For this review, take the finished solid that the model builds, in its own axes (mm). Round coordinates to 2 decimals unless told otherwise and drop trailing zeros. Write each loop counter-clockwise with the first axis right and the second up, starting at its lowest first coordinate (ties: lowest second). Pieces come first, ordered by that corner, then holes. Notation, with made-up numbers: (2.5, 0.25) -> (61.5, 0.25) arc R5 cw to (61.5, 7.25) -> close; hole circle Ø8 at (3, -5.75). An arc over 180 degrees is marked (long way). Answer in a Markdown table with one row per item.
from build123d import *

# Parameters (mm, degrees)
F0_R     = 4
F0_R_2   = 2.5
F0_R_3   = 1.5
F1_DEPTH = 3
F2_DEPTH = 3
F3_R     = 0.6
F4_R     = 2


with BuildPart() as f1:
    # F0 (on Top) → F1 (new body)
    with BuildSketch(Plane.XY):
        Circle(F0_R)
        Circle(F0_R_2, mode=Mode.SUBTRACT)
        Circle(F0_R_2)
        Circle(F0_R_3, mode=Mode.SUBTRACT)
    extrude(amount=F1_DEPTH)

    # F0 (on Top) → F2 (join)
    with BuildSketch(Plane.XY):
        Circle(F0_R_2)
        Circle(F0_R_3, mode=Mode.SUBTRACT)
    extrude(amount=-F2_DEPTH)

    # F3
    f3_edges = [f1.edges().sort_by_distance(p)[0] for p in [
        (-1.5, 0, -3),
    ]]
    fillet(f3_edges, radius=F3_R)

    # F4
    f4_edges = [f1.edges().sort_by_distance(p)[0] for p in [
        (-1.5, 0, 3),
    ]]
    fillet(f4_edges, radius=F4_R)


solid = f1.part
1) Consider section A-A on y = 0. State the section outline as (x, z) points, then the cut area to 3 significant figures.
Solved:
| item | result |
|---|---|
| outline | (-4, 0) -> (-2.5, 0) -> (-2.5, -3) -> (-2.1, -3) arc R0.6 ccw to (-1.5, -2.4) -> (-1.5, 1) arc R2 ccw to (-3.5, 3) -> (-4, 3) -> close; (1.5, -2.4) arc R0.6 ccw to (2.1, -3) -> (2.5, -3) -> (2.5, 0) -> (4, 0) -> (4, 3) -> (3.5, 3) arc R2 ccw to (1.5, 1) -> close |
| area | 19.1 mm² |
2) Clearance check with flat-ended pins moving along their axes: pin 1 Ø1 at (y, z) = (2.5, 2) entering from -X; pin 2 Ø2 at (y, z) = (0, -1.5) entering from +X; pin 3 Ø1 at (y, z) = (1, 2.5) entering from -X; pin 4 Ø3 at (x, z) = (-0.5, 0.5) entering from -Y. State where each tip first meets the part, or that it passes through.
Solved:
| item | result |
|---|---|
| pin 1 | x = -3.46 |
| pin 2 | x = 2.5 |
| pin 3 | x = -3.97 |
| pin 4 | y = -4 |
3) Consider section D-D on y = 3.75. State the section outline as (x, z) points.
Solved:
| item | result |
|---|---|
| outline | (-1.39, 0) -> (1.39, 0) -> (1.39, 3) -> (-1.39, 3) -> close |
4) Mouldability with a two-part tool opening along X and no side actions: class faces 1 (the cylindrical face through (-0.54, -2.44, -1.48)), 2 (the cylindrical face through (-1.5, 0.07, -0.72)), 3 (the flat face through (2, 2, 0)) as pulls with the +X half, pulls with the -X half, needs draft (parallel to the pull), parting line crosses it, or undercut.
Solved:
| item | result |
|---|---|
| face 1 | parting line crosses it |
| face 2 | undercut |
| face 3 | needs draft |
5) Consider section C-C on z = -1.2. State the section outline as (x, y) points.
Solved:
| item | result |
|---|---|
| outline | circle Ø5 at (0, 0); hole circle Ø3 at (0, 0) |
6) For line 1 (Y direction, x = 0, z = -0.2); line 2 (Y direction, x = 0, z = 0.2); line 3 (Y direction, x = 2, z = -1.1), list the stretches that pass through material, from the lowest coordinate up. Write a range as [from, to].
Solved:
| item | result |
|---|---|
| line 1 | [-2.5, -1.5], [1.5, 2.5] |
| line 2 | [-4, -1.5], [1.5, 4] |
| line 3 | [-1.5, 1.5] |
